For this review, take the finished solid that the model builds, in its own axes (mm). A direction names the side the tool comes from. Give positions to 0.01 mm unless a question says otherwise; leave off trailing zeros. Loops run counter-clockwise (first coordinate to the right, second up) from the corner with the lowest first, then second, coordinate; pieces in that order, holes last.
```python
from build123d import *

# Parameters (mm, degrees)
SKETCH_W          = 138
SKETCH_H          = 10
PAD_DEPTH         = 10
SKETCH001_W       = 10
SKETCH001_H       = 10
PAD001_DEPTH      = 100
SKETCH002_R       = 8
PAD002_DEPTH      = 11
PAD002_DEPTH_BACK = 149


with BuildPart() as part:
    # Sketch → Pad (new body)
    with BuildSketch(Plane(origin=(0, 0, 110), x_dir=(1, 0, 0), z_dir=(0, 0, -1))):
        Rectangle(SKETCH_W, SKETCH_H)
    extrude(amount=PAD_DEPTH)

    # Sketch001 → Pad001 (new body)
    with BuildSketch(Plane(origin=(0, 0, 100), x_dir=(1, 0, 0), z_dir=(0, 0, -1))):
        with Locations((-64, 0)):
            Rectangle(SKETCH001_W, SKETCH001_H)
    pad001 = extrude(amount=PAD001_DEPTH)

    # Mirrored: Pad001 across Sketch001 V_Axis
    add(pad001.mirror(Plane(origin=(0, 0, 100), x_dir=(0, 0, -1), z_dir=(1, 0, 0))))

    # Sketch002 → Pad002 (new body, two sides)
    with BuildSketch(Plane(origin=(-69, 0, 110), x_dir=(0, 1, 0), z_dir=(-1, 0, 0))) as pad002_sk:
        with Locations((0, 110)):
            Circle(SKETCH002_R)
    extrude(amount=PAD002_DEPTH)
    extrude(pad002_sk.sketch, amount=-PAD002_DEPTH_BACK)


solid = part.part
```
Q1. For pin 1 Ø2 at (y, z) = (1.5, 26.5) entering from -X; pin 2 Ø8 at (y, z) = (6, 23) entering from +X, all flat-tipped, find the tip position at first contact; note any pin that passes through.
Answers:
pin 1: stops at x = -69
pin 2: stops at x = 69
Q2. Machinability: for faces 1 (the flat face through (0, -5, 101)), 2 (the flat face through (-1, 0, 100)), 3 (the flat face through (-80, 0, 0)), which of the approach directions +Z, -Z, +X, -X, +Y, -Y give a long, thin tool a straight path to every point of the face, cutting with its end or side? Answer none if there is none.
Answers:
face 1: +Z, +X, -X, -Y
face 2: +Y, -Y
face 3: +Z, -Z, -X, +Y, -Y
Q3. For probe 1 along X at (y, z) = (0.75, 10); probe 2 along Y at (x, z) = (12.5, 102); probe 3 along Y at (x, z) = (-56, -0.5), list the stretches that pass through material, from the lowest coordinate up.
Answers:
probe 1: x = -69 to -59, 59 to 69
probe 2: y = -5 to 5
probe 3: y = -7.98 to 7.98
Q4. Mouldability with a two-part tool opening along X and no side actions: class faces 4 (the flat face through (80, 0, 0)), 5 (the flat face through (-59, 0, 54)), 6 (the flat face through (0, 5, 101)) as +X half, -X half, draft (parallel to the pull), parting line (faces both ways), or undercut.
Answers:
face 4: +X half
face 5: undercut
face 6: draft
Q5. Consider section C-C on x = 13. Give the boundary of the cut face in (y, z).
Answers:
outline: circle Ø16 at (0, 0); (-5, 100) - (5, 100) - (5, 110) - (-5, 110) - close
Q6. Consider section B-B on y = 0. Give the boundary of the cut face in (x, z).
Answers:
outline: (-80, -8) - (80, -8) - (80, 8) - (69, 8) - (69, 110) - (-69, 110) - (-69, 8) - (-80, 8) - close; hole (-59, 8) - (59, 8) - (59, 100) - (-59, 100) - close
Q7. Consider section A-A on z = 66. Give the boundary of the cut face in (x, y), plus the area to 3 significant figures.
Answers:
outline: (-69, -5) - (-59, -5) - (-59, 5) - (-69, 5) - close; (59, -5) - (69, -5) - (69, 5) - (59, 5) - close
area: 200 mm2
